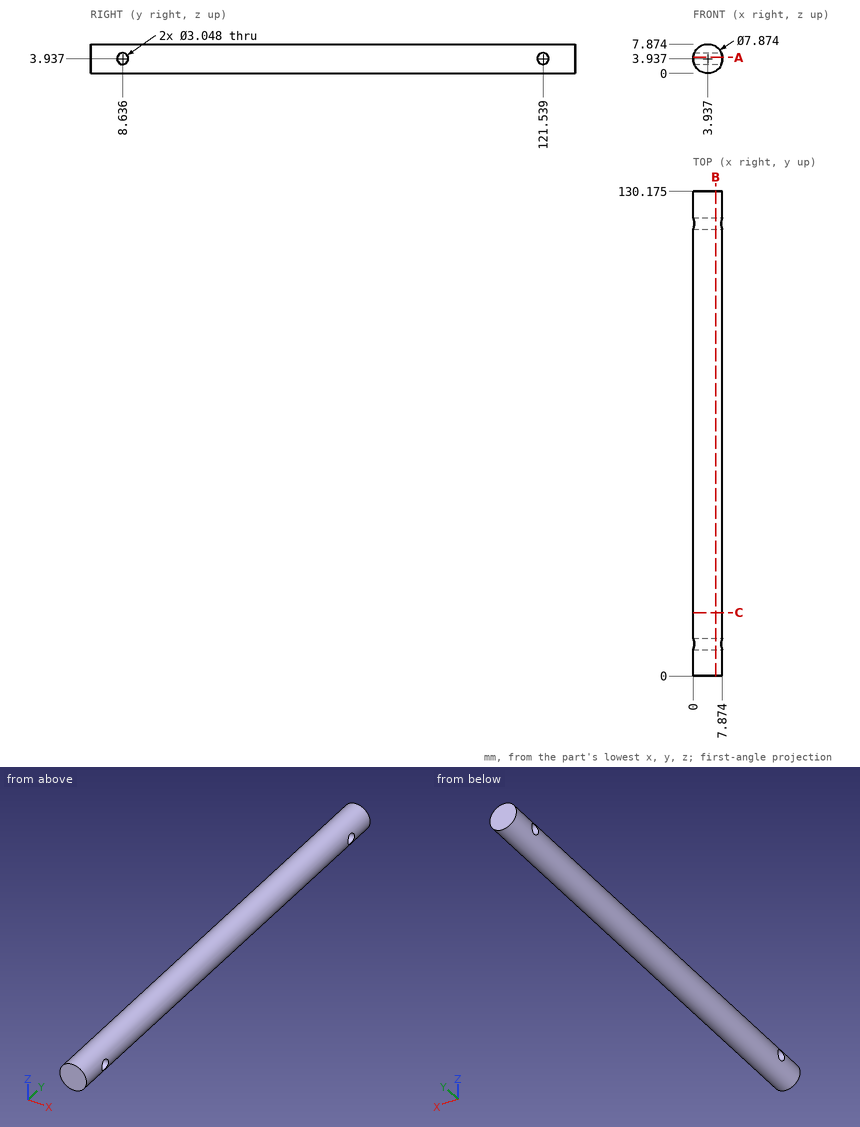
Part print with two shaded views. Sizes in mm from the minimum x, y, z corner. Coordinates: 2 decimals unless noted, no trailing zeros. Write each loop counter-clockwise with the first axis right and the second up, starting at its lowest first coordinate (ties: lowest second). Pieces come first, ordered by that corner, then holes. Notation, with made-up numbers: (-37.5, 7.5) - (13.5, 7.5) arc R26 cw to (13.5, 31.5) - close; hole circle Ø5 at (-38, 50). An arc over 180 degrees is marked (long way). Put each result on its own line as item: value.
1. Band-saw the part on B-B (x = 6). Write the cut outline in (y, z) (3 decimals).
Final values:
outline: (0, 0.584) - (130.175, 0.584) - (130.175, 7.29) - (0, 7.29) - close; hole circle Ø3.048 at (8.636, 3.937); hole circle Ø3.048 at (121.539, 3.937)
2. Band-saw the part on C-C (y = 17). Write the cut outline in (x, z), then the cut area to 3 significant figures.
Final values:
outline: circle Ø7.87 at (3.94, 3.94)
area: 48.7 mm²
3. Band-saw the part on A-A (z = 4.25). Write the cut outline in (x, y) (3 decimals), then the cut area to 3 significant figures.
Final values:
outline: (0.012, 0) - (7.862, 0) - (7.862, 7.144) - (0.012, 7.144) - close; (0.012, 10.128) - (7.862, 10.128) - (7.862, 120.047) - (0.012, 120.047) - close; (0.012, 123.031) - (7.862, 123.031) - (7.862, 130.175) - (0.012, 130.175) - close
area: 975 mm²
4. Flat gauge pins, fed straight in: pin 1 Ø3 at (x, y) = (6, 80.5) entering from -Z; pin 2 Ø1 at (x, y) = (6, 113.5) entering from -Z. Where does each tip first touch, or does it go through?
Final values:
pin 1: stops at z = 0.04
pin 2: stops at z = 0.32
5. Probe line 1 along Y through (x, z) = (1, 4) (3 decimals); line 2 along Y through (x, z) = (2.5, 4.5) (3 decimals); line 3 along Z through (x, y) = (3.5, 94). List the from-to ranges inside material, lowest first. Write a range as [from, to].
Final values:
line 1: y = [0, 7.113], [10.159, 120.016], [123.062, 130.175]
line 2: y = [0, 7.22], [10.052, 120.123], [122.955, 130.175]
line 3: z = [0.02, 7.85]
